Read the model definition and answer for the solid it produces. Units are mm, in the model's axes. A direction names the side the tool comes from. Coordinates: 2 decimals unless noted, no trailing zeros. Order: outer loops, then holes, each group sorted by start corner. A loop starts at its lowest first (then second) coordinate and runs counter-clockwise, first axis right, second up.
```python
from build123d import *

# Parameters (mm, degrees)
FILLET_R     = 0.2
POCKET_DEPTH = 1.3
FILLET001_R  = 0.2


with BuildPart() as part:
    # Sketch → Revolution (revolve)
    with BuildSketch(Plane.XY):
        Polygon((0, 0), (0, 12), (2.7, 12), (2.7, 10), (1.5, 10), (1.5, 0), align=None)
    revolve(axis=Axis((0, 0, 0), (0, 1, 0)))

    # Fillet
    fillet_edges = [part.edges().sort_by_distance(p)[0] for p in [
        (-2.7, 10, 0),
        (-2.7, 12, 0),
    ]]
    fillet(fillet_edges, radius=FILLET_R)

    # Sketch001 (on Face1 of Fillet) → Pocket (cut)
    with BuildSketch(Plane(origin=(0, 12, 0), x_dir=(-1, 0, 0), z_dir=(0, 1, 0))):
        Polygon((0.5, 1.5), (0.5, 0.5), (1.5, 0.5), (1.5, -0.5), (0.5, -0.5), (0.5, -1.5), (-0.5, -1.5), (-0.5, -0.5), (-1.5, -0.5), (-1.5, 0.5), (-0.5, 0.5), (-0.5, 1.5), align=None)
    extrude(amount=-POCKET_DEPTH, mode=Mode.SUBTRACT)

    # Fillet001
    fillet001_edges = [part.edges().sort_by_distance(p)[0] for p in [
        (0, 12, -1.5),
        (0.5, 12, -1),
        (1, 12, -0.5),
        (1.5, 12, 0),
        (1, 12, 0.5),
        (0.5, 12, 1),
        (-0.5, 12, 1),
        (0, 12, 1.5),
        (-1.5, 12, 0),
        (-1, 12, -0.5),
        (-0.5, 12, -1),
    ]]
    fillet(fillet001_edges, radius=FILLET001_R)


solid = part.part
```
1) A cutting plane is placed at B-B, the plane x = 0. Determine the outline of the cut face in (y, z).
A:
outline: (0, -1.5) - (10, -1.5) - (10, -2.5) arc R0.2 ccw to (10.2, -2.7) - (11.8, -2.7) arc R0.2 ccw to (12, -2.5) - (12, -1.7) arc R0.2 ccw to (11.8, -1.5) - (10.7, -1.5) - (10.7, 1.5) - (11.8, 1.5) arc R0.2 ccw to (12, 1.7) - (12, 2.5) arc R0.2 ccw to (11.8, 2.7) - (10.2, 2.7) arc R0.2 ccw to (10, 2.5) - (10, 1.5) - (0, 1.5) - close
2) Determine the mould class of faces 1 (the cylindrical face through (-1.5, 4.93, -0.07)), 2 (the flat face through (0, 0, 0)), 3 (the flat face through (-0.5, 11, -1)), 4 (the flat face through (-1, 11, 0.5)) for opening direction X: pulls with the +X half, pulls with the -X half, needs draft (parallel to the pull), parting line crosses it, or undercut.
A:
face 1: parting line crosses it
face 2: needs draft
face 3: undercut
face 4: undercut
3) Straight lines are drawn through the part: line 1 (Y direction, x = 1.8, z = 0.55); line 2 (Y direction, x = -0.2, z = 0.6); line 3 (Z direction, x = 0.4, y = 11.25). For each, find the intervals that lie inside material, in ascending order.
A:
line 1: y = 10 to 12
line 2: y = 0 to 10.7
line 3: z = -2.67 to -1.5, 1.5 to 2.67
4) A cutting plane is placed at D-D, the plane y = 3.5. Determine the outline of the cut face in (x, z), and give its area (3 significant figures).
A:
outline: circle Ø3 at (0, 0)
area: 7.07 mm2
5) A cutting plane is placed at C-C, the plane z = 0. Determine the outline of the cut face in (x, y), and give its area (3 significant figures).
A:
outline: (-2.7, 10.2) arc R0.2 ccw to (-2.5, 10) - (-1.5, 10) - (-1.5, 0) - (1.5, 0) - (1.5, 10) - (2.5, 10) arc R0.2 ccw to (2.7, 10.2) - (2.7, 11.8) arc R0.2 ccw to (2.5, 12) - (1.7, 12) arc R0.2 ccw to (1.5, 11.8) - (1.5, 10.7) - (-1.5, 10.7) - (-1.5, 11.8) arc R0.2 ccw to (-1.7, 12) - (-2.5, 12) arc R0.2 ccw to (-2.7, 11.8) - close
area: 36.8 mm2
6) Which of the six approach directions +Z, -Z, +X, -X, +Y, -Y give full straight-line access (tool end or side, diameter ignored) to faces 5 (the cylindrical face through (-0.585, 10.989, 2.636)), 6 (the flat face through (2, 10, 0)), 7 (the flat face through (0.5, 11, -1))?
A:
face 5: +Y, -Y
face 6: -Y
face 7: +Y
7) A cutting plane is placed at A-A, the plane y = 11.25. Determine the outline of the cut face in (x, z), and give its area (3 significant figures).
A:
outline: circle Ø5.4 at (0, 0); hole (-1.5, -0.5) - (-0.5, -0.5) - (-0.5, -1.5) - (0.5, -1.5) - (0.5, -0.5) - (1.5, -0.5) - (1.5, 0.5) - (0.5, 0.5) - (0.5, 1.5) - (-0.5, 1.5) - (-0.5, 0.5) - (-1.5, 0.5) - close
area: 17.9 mm2
8) Flat-ended cylindrical pins translate along their axes: pin 1 Ø1.1 at (y, z) = (11.5, -1) entering from -X; pin 2 Ø0.8 at (y, z) = (11.5, 1) entering from -X; pin 3 Ø1.1 at (y, z) = (11, -1) entering from +X. Find the tip coordinate at first contact, or state that the pin passes through.
A:
pin 1: stops at x = -2.66
pin 2: stops at x = -2.63
pin 3: stops at x = 2.66
